Could you check a few things on this model? Use its own coordinates, in mm. Face numbers are marked on the shaded views. A direction names the side the tool comes from. Give positions to 0.01 mm unless a question says otherwise; leave off trailing zeros. Loops run counter-clockwise (first coordinate to the right, second up) from the corner with the lowest first, then second, coordinate; pieces in that order, holes last. Notation, with made-up numbers: (11, -19.75) -> (34, -19.75) arc R37 ccw to (34, 18.25) -> close; hole circle Ø6 at (10.5, 60.25). An arc over 180 degrees is marked (long way). Write each question's results on one line, items separated by ' | '. Start each with the question number.
Q1. Which directions (+Z, -Z, +X, -X, +Y, -Y) give clear straight access to the entire face, cutting with the end or side of a thin tool? Please do the marked faces 1 and 2.
Q2. Will these pins go through, and if not, where does the flat tip stop? P1, Ø1.5, axis at y = 12.5, z = -8.5, coming from the -X side; P2, Ø5, axis at x = -3, y = 18, coming from the -Z side; P3, Ø3, axis at y = 5, z = 12.5, coming from the +X side; P4, Ø2, axis at x = -51.5, z = 2, coming from the -Y side.
Q3. If I drill on line 1 along Z through (x, y) = (-43.5, 2.5); line 2 along X through (y, z) = (27, 0), over which ranges is the centre line in solid material (lowest first)?
Q4. We'd pull the mould along Y, two halves only. Please class the marked faces 3, 4 and 5: released by +Y, released by -Y, zero draft, split by the parting line, or undercut.
Q5. If we section it at B-B, the plane z = -7: List the corners of the cut face in (x, y) for me, plus the area to 3 significant figures.
Q6. If we section it at A-A, the plane x = -29: List the corners of the cut face in (y, z) for me.
Q7. If we section it at D-D, the plane x = -6: List the corners of the cut face in (y, z) for me.
Q8. If we section it at C-C, the plane y = 17.5: List the corners of the cut face in (x, z) for me, plus the area to 3 significant figures.
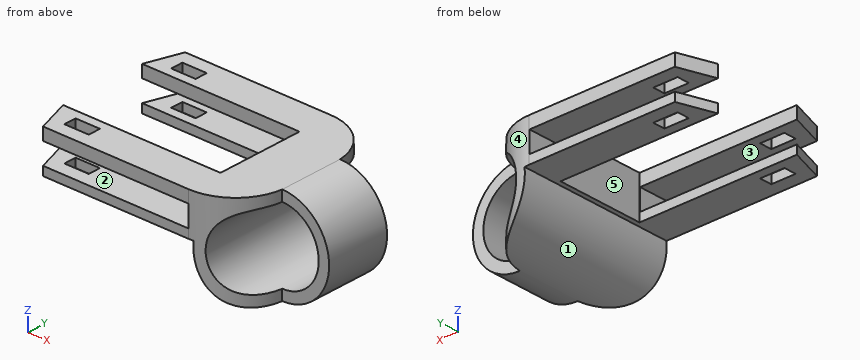
Autodesk Inventor part; units mm, degrees
ref_plane "YZ Plane" through (0, 0, 0) normal (1, 0, 0) x (0, 1, 0)
ref_plane "XZ Plane" through (0, 0, 0) normal (0, 1, 0) x (-1, 0, 0)
ref_plane "XY Plane" through (0, 0, 0) normal (0, 0, 1) x (1, 0, 0)
sketch "Sketch1" plane through (0, 0, 0) normal (0, 1, 0) x (-1, 0, 0)
  circle A0 centre (0, 0) radius 10.5
  arc A1 (0, 13.5) -> (13.4164, 1.5) centre (0, 0) ccw
  line L0 (0, 13.5) -> (60, 13.5)
  line L1 (60, 13.5) -> (60, 1.5)
  line L2 (60, 1.5) -> (13.4164, 1.5)
  dimension "d1" = 21
  dimension "d2" = 60
  dimension "d3" = 12
  dimension "d6" = 3
extrude "Extrusion1" add sketch "Sketch1" along normal blind 45
sketch "Sketch2" plane through (-60, 0, 13.5) normal (0, 0, 1) x (1, 0, 0)
  line L0 (0, 45) -> (60, 45)
  line L1 (0, 35) -> (3.306, 45)
  line L2 (51.1457, 45) -> (3.306, 45)
  line L3 (0, 35) -> (45.2583, 35)
  line L4 (0, 22.5) -> (103.0931, 22.5) construction
  line L5 (0, 0) -> (60, 0)
  line L6 (0, 10) -> (3.306, 0)
  line L7 (0, 10) -> (45.2583, 10)
  line L8 (45.2583, 35) -> (45.2583, 10)
  line L9 (0, 35) -> (0, 10)
  line L10 (60, 0) -> (60, 45)
  line L11 (0, 10) -> (0, 0)
  line L12 (0, 0) -> (60, 0)
  line L13 (0, 45) -> (0, 35)
  line L14 (3.306, 45) -> (0, 45)
extrude "Extrusion2" cut sketch "Sketch2" against normal blind 12 contours L0 L1 L13 | L3 L8 L7 L9 | L6 L5 L11
sketch "Sketch3" plane through (0, 45, 0) normal (0, 1, 0) x (1, 0, 0)
  line L0 (-60, -1.5) -> (-60, -13.5)
  line L1 (-60, -4) -> (-14.8943, -4)
  line L2 (-14.8943, -4) -> (-14.8943, -10)
  line L3 (-14.8943, -10) -> (-60, -10)
  line L4 (-60, -4) -> (-60, -10)
extrude "Extrusion3" cut sketch "Sketch3" against normal blind 45
sketch "Sketch4" plane through (0, 0, 13.5) normal (0, 0, 1) x (1, 0, 0)
  line L0 (-56.694, 0) -> (0, 0)
  line L1 (0, 0) -> (0, 45)
  line L2 (-56.694, 45) -> (0, 45)
  arc A0 (0, 31.6668) -> (-14.7825, 45) centre (-14.7825, 30.1387) ccw
  line L3 (0, 31.6668) -> (14.4337, 31.6668)
  line L4 (-19.4308, 22.5) -> (16.7273, 22.5) construction
  line L5 (14.4337, 31.6668) -> (14.4337, 22.5)
  line L6 (0, 13.3332) -> (14.4337, 13.3332)
  line L7 (14.4337, 13.3332) -> (14.4337, 22.5)
  arc A1 (-14.7825, 0) -> (0, 13.3332) centre (-14.7825, 14.8613) ccw
  line L8 (-14.7825, 45) -> (14.4337, 45)
  line L9 (14.4337, 45) -> (14.4337, 31.6668)
  line L10 (14.4337, 13.3332) -> (14.4337, 0)
  line L11 (14.4337, 0) -> (-14.7825, 0)
extrude "Extrusion4" cut sketch "Sketch4" against normal blind 45 contours A1 L1 L0 | L1 L6 L10 L11 | A0 L2 L1 | L1 L8 L9 L3
sketch "Sketch5" plane through (-60, 35, 13.5) normal (0, 0, 1) x (1, 0, 0)
  line L0 (45.2583, 0) -> (45.2583, -25)
  line L1 (12.9797, 6.1743) -> (5.9797, 6.1743)
  line L2 (5.9797, 6.1743) -> (5.9797, 2.6291)
  line L3 (5.9797, 2.6291) -> (12.9797, 2.6291)
  line L4 (12.9797, 2.6291) -> (12.9797, 6.1743)
  line L5 (45.2583, -12.5) -> (-11.096, -12.5) construction
  line L6 (12.9797, -31.1743) -> (5.9797, -31.1743)
  line L7 (5.9797, -31.1743) -> (5.9797, -27.6291)
  line L8 (5.9797, -27.6291) -> (12.9797, -27.6291)
  line L9 (12.9797, -27.6291) -> (12.9797, -31.1743)
  point P0 (60, -35)
  dimension "d16" = 7
extrude "Extrusion5" cut sketch "Sketch5" against normal blind 15
properties part number "soporte camara"
Final values:
1) face 1: +Y, -Y | face 2: -X, +Y, -Y
2) P1: stops at x = -11.05 | P2: stops at z = -13.49 | P3: stops at x = -2.5 | P4: stops at y = 0
3) line 1: z = 1.5 to 4, 10 to 13.5 | line 2: x = -13.5 to -10.5, 10.5 to 13.5
4) face 3: zero draft | face 4: released by +Y | face 5: undercut
5) outline: (-11.54, 0.36) arc R14.86 ccw to (-7.83, 1.73) -> (-7.83, 43.27) arc R14.86 ccw to (-11.54, 44.64) -> close; (7.83, 13.33) -> (11.54, 13.33) -> (11.54, 31.67) -> (7.83, 31.67) -> close | area: 228 mm²
6) outline: (0, 1.5) -> (10, 1.5) -> (10, 4) -> (0, 4) -> close; (0, 10) -> (10, 10) -> (10, 13.5) -> (0, 13.5) -> close; (35, 1.5) -> (45, 1.5) -> (45, 4) -> (35, 4) -> close; (35, 10) -> (45, 10) -> (45, 13.5) -> (35, 13.5) -> close
7) outline: (2.87, -12.09) -> (42.13, -12.09) -> (42.13, -8.62) -> (2.87, -8.62) -> close; (2.87, 8.62) -> (42.13, 8.62) -> (42.13, 13.5) -> (2.87, 13.5) -> close
8) outline: (-14.74, 1.5) -> (-13.42, 1.5) arc R13.5 ccw (long way) to (0, 13.5) -> (-14.74, 13.5) -> close; hole circle Ø21 at (0, 0) | area: 280 mm²
